Work out the finished part from the listing and answer in its coordinate system (mm). Face numbers are marked on the shaded views. Round coordinates to 2 decimals unless told otherwise and drop trailing zeros. Order: outer loops, then holes, each group sorted by start corner. A loop starts at its lowest first (then second) coordinate and runs counter-clockwise, first axis right, second up. Notation, with made-up numbers: (38, 64.5) -> (94, 64.5) arc R15 ccw to (94, 82.5) -> close; hole circle Ø9 at (63.5, -36). An arc over 180 degrees is marked (long way). Use a Markdown table: item, result. Add a question column.
Item 1: For a pull along Y with two mould halves and no side action, classify the marked faces 1, 2 and 3 as +Y half, -Y half, draft (parallel to the pull), parting line (faces both ways), or undercut.
Item 2: Flat-ended cylindrical pins translate along their axes: P1, Ø4.5, axis at x = 0, y = 10.06, coming from the +Z side; P2, Ø4.5, axis at y = 65.5, z = 5.5, coming from the -X side; P3, Ø3, axis at y = 64.5, z = 5, coming from the +X side. Find the tip coordinate at first contact, or state that the pin passes through.
Item 3: Find the intervals of material crossed by L1, parallel to Y at x = 0, z = 14; L2, parallel to Y at x = 0, z = 17.25; L3, parallel to Y at x = -0.75, z = 5, in increasing order. Write a range as [from, to].
Item 4: A cutting plane is placed at D-D, the plane y = 63.5. Determine the outline of the cut face in (x, z) (3 decimals).
Item 5: A cutting plane is placed at C-C, the plane z = 12.75. Determine the outline of the cut face in (x, y), plus the area to 3 significant figures.
Item 6: A cutting plane is placed at A-A, the plane y = 79.5. Determine the outline of the cut face in (x, z), plus the area to 3 significant figures.
Item 7: A cutting plane is placed at B-B, the plane z = 4.5. Determine the outline of the cut face in (x, y).
Autodesk Inventor part; units mm, degrees
ref_plane "Work Plane2" through (-88.5, 89.5, 29.5) normal (0, 0, 1) x (1, 0, 0)
ref_plane "YZ Plane" through (0, 0, 0) normal (1, 0, 0) x (0, 1, 0)
ref_plane "XZ Plane" through (0, 0, 0) normal (0, 1, 0) x (-1, 0, 0)
ref_plane "Work Plane1" through (0, 0, 0) normal (0, 0, 1) x (1, 0, 0)
sketch "Sketch1" plane through (0, 0, 0) normal (0, 0, 1) x (1, 0, 0)
  line L0 (-74, -73.5) -> (-74, -89.5)
  line L1 (-74, -89.5) -> (74, -89.5)
  line L2 (74, -89.5) -> (74, -73.5)
  line L3 (74, -73.5) -> (89, -73.5)
  line L4 (89, -73.5) -> (89, 37.5)
  line L5 (89, 37.5) -> (22.5, 37.5)
  line L6 (22.5, 37.5) -> (22.5, 89.5)
  line L7 (22.5, 89.5) -> (16.5, 89.5)
  line L8 (16.5, 89.5) -> (16.5, 37.5)
  line L9 (16.5, 37.5) -> (4.5, 37.5)
  line L10 (4.5, 37.5) -> (4.5, 89.5)
  line L11 (4.5, 89.5) -> (-4.5, 89.5)
  line L12 (-4.5, 89.5) -> (-4.5, 37.5)
  line L13 (-4.5, 37.5) -> (-16.5, 37.5)
  line L14 (-16.5, 37.5) -> (-16.5, 89.5)
  line L15 (-16.5, 89.5) -> (-22.5, 89.5)
  line L16 (-22.5, 89.5) -> (-22.5, 37.5)
  line L17 (-22.5, 37.5) -> (-89, 37.5)
  line L18 (-89, 37.5) -> (-89, -73.5)
  line L19 (-89, -73.5) -> (-74, -73.5)
  circle A0 centre (-29.2, 3.1615) radius 1.8
  line L20 (-22.5, 13.4539) -> (-22.5, 0.9615)
  line L21 (-27.2, 13.4539) -> (-22.5, 13.4539)
  line L22 (-27.2, 13.4539) -> (-27.2, 5.7703)
  line L23 (-27.2, 5.7703) -> (-32.2, 5.7703)
  line L24 (-32.2, 0.9615) -> (-32.2, 5.7703)
  line L25 (-32.2, 0.9615) -> (-22.5, 0.9615)
  circle A1 centre (29.2, 3.1615) radius 1.8
  line L26 (22.5, 13.4539) -> (22.5, 0.9615)
  line L27 (32.2, 0.9615) -> (22.5, 0.9615)
  line L28 (32.2, 0.9615) -> (32.2, 5.7703)
  line L29 (27.2, 5.7703) -> (32.2, 5.7703)
  line L30 (27.2, 13.4539) -> (27.2, 5.7703)
  line L31 (27.2, 13.4539) -> (22.5, 13.4539)
  line L32 (-4.5, 89.5) -> (4.5, 89.5)
  line L33 (4.5, 89.5) -> (4.5, 0.9615)
  line L34 (4.5, 0.9615) -> (-4.5, 0.9615)
  line L35 (-4.5, 0.9615) -> (-4.5, 89.5)
  point P0 (0, 0)
ref_plane "Work Plane2" through (-88.5, 89.5, 29.5) normal (0, 0, 1) x (1, 0, 0)
extrude "Extrusion1" add sketch "Sketch1" along normal up to surface (29.5 mm away) contours L12 L11 L10 L33 L34 L35
sketch "Sketch2" plane through (4.5, 0.9615, 0) normal (1, 0, 0) x (0, 0, -1)
  circle A0 centre (-16.1803, 34.1432) radius 2
  point P0 (0, -0.9615)
extrude "Extrusion2" cut sketch "Sketch2" against normal up to next
sketch "Sketch3" plane through (4.5, 0.9615, 0) normal (1, 0, 0) x (0, 0, -1)
  circle A0 centre (-6.5, 62.5385) radius 5.5
  circle A1 centre (-6.5, 62.5385) radius 4.5
  circle A2 centre (-6.5, 62.5385) radius 4.65
  point P0 (0, -0.9615)
  dimension "d4" = 9
  dimension "d5" = 0.15
extrude "Extrusion3" cut sketch "Sketch3" against normal blind 4.3 contours A1 | A2
sketch "Sketch4" plane through (-4.5, 0.9615, 0) normal (-1, 0, 0) x (0, 0, 1)
  circle A0 centre (6.5, 62.5385) radius 1.2295
  circle A1 centre (6.5, 62.5385) radius 4.65
  circle A2 centre (6.5, 62.5385) radius 4.575
  point P0 (0, -0.9615)
  dimension "d8" = 9.15
extrude "Extrusion4" cut sketch "Sketch4" against normal blind 4.3 contours A0 | A2
sketch "Sketch6" plane through (-4.5, 0.9615, 0) normal (-1, 0, 0) x (0, 0, 1)
  circle A0 centre (5, 20) radius 1.8
  circle A1 centre (23.5, 78.5385) radius 1.8
  point P0 (0, -0.9615)
extrude "Extrusion5" cut sketch "Sketch6" against normal up to surface (9 mm away)
sketch "Sketch7" plane through (-4.5, 0.9615, 29.5) normal (0, 0, 1) x (1, 0, 0)
  line L0 (9, 21.8) -> (9, 18.2)
  line L1 (0, 18.2) -> (0, 21.8)
  line L2 (0, 32.1432) -> (0, 36.1432)
  line L3 (9, 36.1432) -> (9, 32.1432)
  line L4 (4.3, 57.9635) -> (4.3, 67.1135)
  line L5 (0, 57.9635) -> (0, 67.1135)
  line L6 (0, 76.7385) -> (0, 80.3385)
  line L7 (9, 88.5385) -> (9, 0)
  line L8 (0, 80.3385) -> (9, 80.3385)
  line L9 (9, 80.3385) -> (9, 76.7385)
  line L10 (9, 76.7385) -> (0, 76.7385)
  line L11 (0, 76.7385) -> (0, 80.3385)
  line L12 (9, 57.8885) -> (4.7, 57.8885)
  line L13 (0, 67.1135) -> (9, 67.1135)
  line L14 (9, 67.1135) -> (9, 57.8885)
  line L15 (9, 57.8885) -> (0, 57.8885)
  line L16 (0, 57.8885) -> (0, 67.1135)
  line L17 (0, 36.1432) -> (9, 36.1432)
  line L18 (9, 36.1432) -> (9, 32.1432)
  line L19 (9, 32.1432) -> (0, 32.1432)
  line L20 (0, 32.1432) -> (0, 36.1432)
  line L21 (9, 0) -> (0, 0)
  line L22 (9, 88.5385) -> (9, 0)
  line L23 (0, 88.5385) -> (9, 88.5385)
  line L24 (0, 0) -> (0, 88.5385)
  line L25 (0, 18.2) -> (9, 18.2)
  line L26 (9, 18.2) -> (9, 21.8)
  line L27 (9, 21.8) -> (0, 21.8)
  line L28 (0, 21.8) -> (0, 18.2)
  line L29 (0, 18.2) -> (9, 0)
  line L30 (0, 0) -> (9, 18.2)
  line L31 (9, 36.1432) -> (0, 57.8885)
  line L32 (0, 36.1432) -> (9, 57.8885)
  line L33 (0, 76.7385) -> (9, 67.1135)
  line L34 (0, 67.1135) -> (9, 76.7385)
  point P0 (4.5, -0.9615)
  point P1 (4.5, 9.1)
  point P2 (4.5, 47.0158)
  point P3 (4.5, 71.926)
hole "Hole2" at (0, 10.0615, 29.5) at (0, 47.9774, 29.5) at (0, 72.8875, 29.5) direction (0, 0, -1) diameter 3.6 end through all countersink diameter 6.6 countersink angle 90
properties part number "middle_gaer_holder"
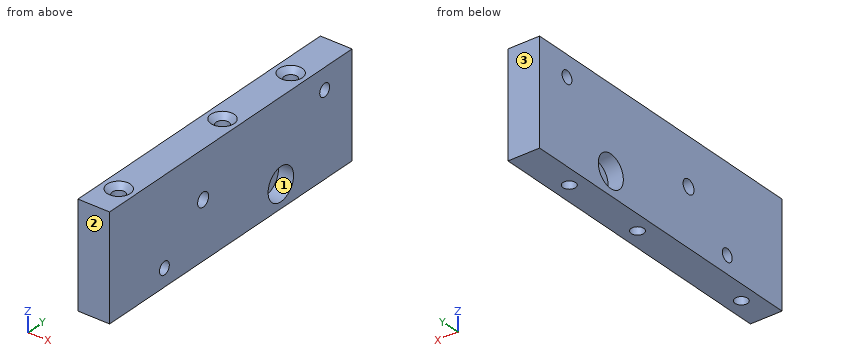
Reported:
| question | item | result |
|---|---|---|
| 1 | face 1 | undercut |
| 1 | face 2 | -Y half |
| 1 | face 3 | +Y half |
| 2 | P1 | z = 28.45 |
| 2 | P2 | x = -0.2 |
| 2 | P3 | x = 0.2 |
| 3 | L1 | [0.96, 8.26], [11.86, 46.18], [49.78, 71.09], [74.69, 89.5] |
| 3 | L2 | [0.96, 8.26], [11.86, 33.41], [36.79, 46.18], [49.78, 71.09], [74.69, 89.5] |
| 3 | L3 | [0.96, 8.43], [11.7, 19.16], [22.76, 46.34], [49.61, 59.18], [67.82, 71.25], [74.52, 89.5] |
| 4 | outline | (-4.5, 0) -> (4.5, 0) -> (4.5, 1.85) -> (0.2, 1.85) -> (0.2, 11.15) -> (4.5, 11.15) -> (4.5, 29.5) -> (-4.5, 29.5) -> (-4.5, 11.075) -> (-0.2, 11.075) -> (-0.2, 1.925) -> (-4.5, 1.925) -> close |
| 5 | outline | (-4.5, 0.96) -> (4.5, 0.96) -> (4.5, 89.5) -> (-4.5, 89.5) -> close; hole circle Ø3.6 at (0, 10.06); hole circle Ø3.6 at (0, 47.98); hole circle Ø3.6 at (0, 72.89) |
| 5 | area | 766 mm² |
| 6 | outline | (-4.5, 0) -> (4.5, 0) -> (4.5, 21.7) -> (-4.5, 21.7) -> close; (-4.5, 25.3) -> (4.5, 25.3) -> (4.5, 29.5) -> (-4.5, 29.5) -> close |
| 6 | area | 233 mm² |
| 7 | outline | (-4.5, 0.96) -> (4.5, 0.96) -> (4.5, 19.23) -> (-4.5, 19.23) -> close; (-4.5, 22.69) -> (4.5, 22.69) -> (4.5, 59.3) -> (0.2, 59.3) -> (0.2, 67.7) -> (4.5, 67.7) -> (4.5, 89.5) -> (-4.5, 89.5) -> (-4.5, 67.61) -> (-0.2, 67.61) -> (-0.2, 59.39) -> (-4.5, 59.39) -> close; hole circle Ø3.6 at (0, 10.06); hole circle Ø3.6 at (0, 47.98); hole circle Ø3.6 at (0, 72.89) |
